Autodesk Inventor part; units mm, degrees
ref_plane "YZ Plane" through (0, 0, 0) normal (1, 0, 0) x (0, 1, 0)
ref_plane "XZ Plane" through (0, 0, 0) normal (0, 1, 0) x (-1, 0, 0)
ref_plane "XY Plane" through (0, 0, 0) normal (0, 0, 1) x (1, 0, 0)
sketch "Szkic1" plane through (0, 0, 0) normal (0, 0, 1) x (1, 0, 0)
  line L0 (0, 0) -> (80, 0)
  line L1 (80, 0) -> (80, 75)
  line L2 (80, 75) -> (0, 75)
  line L3 (0, 75) -> (0, 0)
  circle A0 centre (14, 53.5) radius 3
  line L4 (14, 53.5) -> (14, 21.5)
  circle A1 centre (14, 21.5) radius 3
  line L5 (0, 75) -> (-16, 75)
  line L6 (-16, 75) -> (-16, 0)
  line L7 (-16, 0) -> (0, 0)
  line L8 (0, 0) -> (0, 75)
  dimension "d0" = 80
  dimension "d1" = 75
  dimension "d2" = 6
  dimension "d3" = 32
  dimension "d4" = 6
  dimension "d5" = 16
  dimension "d43" = 66
extrude "Wyciągnięcie proste1" add sketch "Szkic1" along normal blind 4
sketch "Szkic2" plane through (0, 0, 0) normal (0, 0, -1) x (-1, 0, 0)
  line L0 (16, 75) -> (16, 0)
  line L1 (-80, 75) -> (16, 75)
  line L2 (-80, 0) -> (-80, 75)
  line L3 (16, 0) -> (-80, 0)
  circle A0 centre (-14, 53.5) radius 3
  circle A1 centre (-14, 21.5) radius 3
  line L4 (-80, 75) -> (16, 75)
  line L5 (0, 0) -> (-4, 0)
  line L6 (-4, 0) -> (-4, 75)
  line L7 (-4, 75) -> (0, 75)
  line L8 (0, 75) -> (0, 0)
  line L9 (-4, 0) -> (-24, 0)
  line L10 (-24, 0) -> (-24, 75)
  line L11 (-24, 75) -> (-4, 75)
  line L12 (-4, 75) -> (-4, 0)
  line L13 (-24.5, 75) -> (-80.5, 75)
  line L14 (-80.5, 75) -> (-80.5, 13.5)
  line L15 (-80.5, 13.5) -> (-24.5, 13.5)
  line L16 (-24.5, 13.5) -> (-24.5, 75)
  line L17 (-28, 17) -> (-77, 17)
  line L18 (-77, 17) -> (-77, 71.5)
  line L19 (-77, 71.5) -> (-28, 71.5)
  line L20 (-28, 71.5) -> (-28, 17)
  circle A2 centre (-28, 71.5) radius 1
  circle A3 centre (-77, 71.5) radius 1
  circle A4 centre (-28, 71.5) radius 3
  circle A5 centre (-77, 71.5) radius 3
  circle A6 centre (-28, 13.5) radius 1
  circle A7 centre (-77, 13.5) radius 1
  circle A8 centre (-77, 13.5) radius 2.5
  circle A9 centre (-28, 13.5) radius 2.5
  dimension "d8" = 4
  dimension "d9" = 20
  dimension "d10" = 56
  dimension "d11" = 61.5
  dimension "d12" = 3.5
  dimension "d15" = 2
  dimension "d16" = 2
  dimension "d19" = 2
  dimension "d20" = 2
  dimension "d34" = 2
  dimension "d35" = 2
  dimension "d36" = 1.5
  dimension "d37" = 1.5
  dimension "d44" = 4
extrude "Wyciągnięcie proste2" add sketch "Szkic2" along normal blind 3 contours L8 L3 L6 L1 | A5 L19 A3 L18 | A9 L15 A6 | L15 A6 A9 | A8 L15 A7 | L15 A7 A8 | A5 L18 A3 L19 | A4 L20 A2 L19 | L19 A2 L20 A4
sketch "Szkic3" plane through (0, 0, 4) normal (0, 0, 1) x (1, 0, 0)
  circle A0 centre (-14, 37.5) radius 2
  circle A1 centre (-14, 37.5) radius 1
  line L0 (-14, 37.5) -> (57.3, 37.5)
  line L1 (57.3, 37.5) -> (57.3, 53.5)
  line L2 (57.3, 37.5) -> (57.3, 21.5)
  circle A2 centre (57.3, 21.5) radius 1
  circle A3 centre (57.3, 21.5) radius 2
  circle A4 centre (57.3, 53.5) radius 1
  circle A5 centre (57.3, 53.5) radius 2
  point P0 (0, 0)
  dimension "d23" = 4
  dimension "d24" = 2
  dimension "d25" = 71.3
  dimension "d26" = 16
  dimension "d27" = 16
  dimension "d28" = 2
  dimension "d29" = 4
  dimension "d30" = 2
  dimension "d31" = 4
extrude "Wyciągnięcie proste3" add sketch "Szkic3" along normal blind 8
sketch "Szkic4" plane through (0, 0, 4) normal (0, 0, 1) x (1, 0, 0)
  circle A0 centre (28, 71.5) radius 3
  circle A1 centre (77, 13.5) radius 2.5
  circle A2 centre (28, 13.5) radius 2.5
  line L0 (4, 0) -> (4, 75)
  line L1 (80, 75) -> (4, 75)
  line L2 (80, 71.5) -> (80, 75)
  circle A3 centre (77, 71.5) radius 3
  line L3 (80, 0) -> (80, 71.5)
  line L4 (4, 0) -> (80, 0)
  circle A4 centre (14, 53.5) radius 3
  circle A5 centre (14, 21.5) radius 3
  circle A6 centre (57.3, 21.5) radius 2
  circle A7 centre (57.3, 53.5) radius 2
  line L5 (57.3, 23.5) -> (57.3, 51.5)
  line L6 (57.3, 51.5) -> (57.3, 36.5)
  line L7 (57.3, 36.5) -> (80, 36.5)
  arc A8 (57.3, 48.5) -> (57.3, 24.5) centre (57.3, 36.5) ccw
  line L8 (57.3, 24.5) -> (80, 24.5)
  line L9 (57.3, 48.5) -> (80, 48.5)
  point P0 (0, 0)
  dimension "d38" = 15
extrude "Wyciągnięcie proste4" cut sketch "Szkic4" against normal blind 4 contours L8 L5 L7 L3 | L7 L5 L9 L3 | A8 L5
fillet "Zaokrąglenie1" radius 5 2 edges at (80, 24.5, 2) (80, 48.5, 2)
fillet "Zaokrąglenie2" radius 5 2 edges at (0, 37.5, 0) (0, 37.5, -3)
properties part number "RP4_LidarHolder"
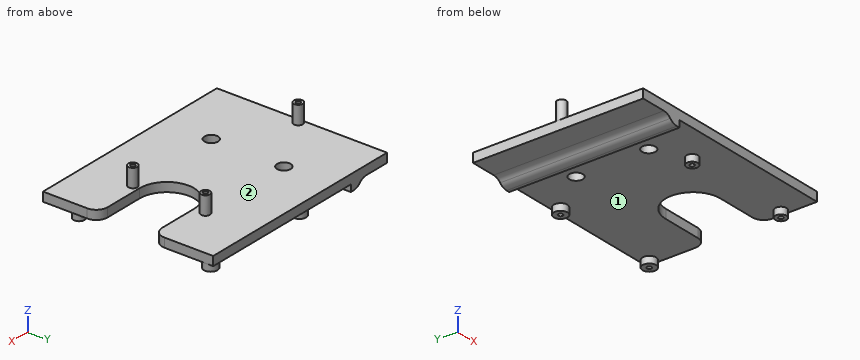
Could you check a few things on this model? Use its own coordinates, in mm. Face numbers are marked on the shaded views. Round coordinates to 2 decimals unless told otherwise and drop trailing zeros. Loops run counter-clockwise (first coordinate to the right, second up) from the corner with the lowest first, then second, coordinate; pieces in that order, holes last. Notation, with made-up numbers: M 86.25,40 L 132.25,40 A5 ccw 132.25,47 Z; hole C -0.5,-9 d10. An arc over 180 degrees is marked long. Write item = value, one per line.
1. Thinking about a two-plate mould opening in Z: for the marked faces 1 and 2, which applies, +Z half, -Z half, draft (parallel to the pull), parting line (faces both ways), or undercut?
Results below:
face_1 = -Z half
face_2 = +Z half
2. I need wall thicknesses on probe 1 along Y at (x, z) = (57.3, 10.5); probe 2 along Y at (x, z) = (-14, 6); probe 3 along X at (y, z) = (53.5, 6). Which ranges of each line are inside material? Lowest first, please.
Results below:
probe_1 = 19.5 to 20.5, 22.5 to 23.5, 51.5 to 52.5, 54.5 to 55.5
probe_2 = 35.5 to 36.5, 38.5 to 39.5
probe_3 = 55.3 to 56.3, 58.3 to 59.3
3. I want a section at B-B, the plane z = 2.75. Write out the boundary of the cut face in (x, y), and give its area (3 significant figures).
Results below:
outline = M -16,0 L 80,0 L 80,19.5 A5 ccw 75,24.5 L 57.3,24.5 A12 cw 57.3,48.5 L 75,48.5 A5 ccw 80,53.5 L 80,75 L -16,75 Z; hole C 14,21.5 d6; hole C 14,53.5 d6
area = 6,360 mm²
4. I want a section at D-D, the plane x = 28. Write out the boundary of the cut face in (y, z), and give its area (3 significant figures).
Results below:
outline = M 0,0 L 11,0 L 11,-3 L 12.5,-3 L 12.5,0 L 14.5,0 L 14.5,-3 L 16,-3 L 16,0 L 68.5,0 L 68.5,-3 L 70.5,-3 L 70.5,0 L 72.5,0 L 72.5,-3 L 74.5,-3 L 74.5,0 L 75,0 L 75,4 L 0,4 Z
area = 321 mm²
5. I want a section at C-C, the plane z = 10.25. Write out the boundary of the cut face in (x, y).
Results below:
outline = C -14,37.5 d4; C 57.3,21.5 d4; C 57.3,53.5 d4; hole C -14,37.5 d2; hole C 57.3,21.5 d2; hole C 57.3,53.5 d2
6. I want a section at A-A, the plane x = 65.5. Write out the boundary of the cut face in (y, z), and give its area (3 significant figures).
Results below:
outline = M 0,0 L 24.5,0 L 24.5,4 L 0,4 Z; M 48.5,0 L 75,0 L 75,4 L 48.5,4 Z
area = 204 mm²
7. Will these pins go through, and if not, where does the flat tip stop? P1, Ø3.5, axis at x = -10, y = 50.5, coming from the -Z side; P2, Ø22.5, axis at x = 14, y = 40, coming from the +Z side; P3, Ø6, axis at y = 42.5, z = 1.5, coming from the +X side.
Results below:
P1 = 0
P2 = 4
P3 = 49.36
